from build123d import *

# Parameters (mm, degrees)
BOSS_EXTRUDE1_DEPTH = 8


with BuildPart() as part:
    # Sketch1 → Boss-Extrude1 (new body)
    with BuildSketch(Plane(origin=(0, 0, 0), x_dir=(1, 0, 0), z_dir=(0, 1, 0))):
        with BuildLine():
            Line((0, 0), (38, 0))
            ThreePointArc((38, 0), (40.636038969, 6.363961031), (47, 9))
            Line((47, 9), (99, 9))
            ThreePointArc((99, 9), (105.363961031, 6.363961031), (108, 0))
            Line((108, 0), (142, 0))
            Line((142, 0), (172.50354814, 93.880267937))
            ThreePointArc((172.50354814, 93.880267937), (166.569139078, 124.354715336), (137.573015724, 135.451290736))
            Line((137.573015724, 135.451290736), (79.487889635, 127.207214423))
            Line((79.487889635, 127.207214423), (0, 0))
        make_face()
        with BuildLine():
            Line((97.109133521, 75.428206388), (131.785075785, 80.179945877))
            ThreePointArc((131.785075785, 80.179945877), (139.670612135, 74.195105322), (133.68577158, 66.309568971))
            Line((133.68577158, 66.309568971), (99.009829317, 61.557829483))
            ThreePointArc((99.009829317, 61.557829483), (95.579909698, 60.235342824), (93.103530342, 57.518568112))
            ThreePointArc((93.103530342, 57.518568112), (61.402056741, 63.469750476), (90.33394504, 77.729688746))
            ThreePointArc((90.33394504, 77.729688746), (93.449886138, 75.779245046), (97.109133521, 75.428206388))
        make_face(mode=Mode.SUBTRACT)
    extrude(amount=BOSS_EXTRUDE1_DEPTH)


solid = part.part
Check sheet for the modelled part. Datum: model origin and axes. Units: mm. A direction names the side the tool comes from. Round coordinates to 2 decimals unless told otherwise and drop trailing zeros. Order: outer loops, then holes, each group sorted by start corner. A loop starts at its lowest first (then second) coordinate and runs counter-clockwise, first axis right, second up. Notation, with made-up numbers: M -23.75,80.25 L -12.75,80.25 A24 ccw -12.75,90.25 Z; hole C 22.25,-14 d3. An arc over 180 degrees is marked long. One line per item, written item: value. Start each with the question number.
1. Section check B-B on y = 4.25. Enter the section's corners in (x, z).
2. Gauge pin test, flat ends, axial feed: P1, Ø1.5, axis at x = 154.5, y = 3, coming from the -Z side; P2, Ø3, axis at y = 1.5, z = -80, coming from the -X side; P3, Ø2, axis at y = 2, z = -113.5, coming from the +X side. Record the tip position at first contact, or that the pin passes through.
3. Section check A-A on x = 120. Enter the section's corners in (y, z) (3 decimals).
4. Scan lines: line 1 along X through (y, z) = (2.75, -8); line 2 along Z through (x, y) = (121.5, 3.5); line 3 along X through (y, z) = (5.75, -6.5). Record each from-to range of solid material in increasing order.
5. Section check C-C on x = 74.5. Enter the section's corners in (y, z).
6. Access from +Z, -Z, +X, -X, +Y, -Y to the whole of each face (thin tool, end or side, straight path). Record for faces 1 (the cylindrical face through (40.566, 3.944, -6.294)), 2 (the flat face through (125, 4, 0)), 3 (the cylindrical face through (95.623, 3.944, -60.265)).
7. Release check for a two-part mould opening along Z. For faces 4 (the flat face through (105, 0, -54)), 5 (the cylindrical face through (93.401, 3.944, -75.796)), 6 (the flat face through (19, 4, 0)) record: released by +Z, released by -Z, zero draft, split by the parting line, or undercut.
8. Section check D-D on z = -16. Enter the section's corners in (x, y), and give its area (3 significant figures).
Results found:
1. outline: M 0,0 L 79.49,-127.21 L 137.57,-135.45 A32 ccw 172.5,-93.88 L 142,0 L 108,0 A9 cw 99,-9 L 47,-9 A9 cw 38,0 Z; hole M 90.33,-77.73 A8 cw 97.11,-75.43 L 131.79,-80.18 A7 ccw 133.69,-66.31 L 99.01,-61.56 A8 cw 93.1,-57.52 A17 ccw long Z
2. P1: z = -133.56
2. P2: x = 49.05
2. P3: x = 172.86
3. outline: M 0,-132.957 L 8,-132.957 L 8,-78.565 L 0,-78.565 Z; M 0,-64.434 L 8,-64.434 L 8,0 L 0,0 Z
4. line 1: 5 to 42.88, 103.12 to 144.6
4. line 2: -133.17 to -78.77, -64.64 to 0
4. line 3: 4.06 to 40.78, 105.22 to 144.11
5. outline: M 0,-119.22 L 8,-119.22 L 8,-82.36 L 0,-82.36 Z; M 0,-49.2 L 8,-49.2 L 8,-9 L 0,-9 Z
6. face 1: +Z, +Y, -Y
6. face 2: +Z, +X, -X, +Y, -Y
6. face 3: +Y, -Y
7. face 4: zero draft
7. face 5: undercut
7. face 6: released by +Z
8. outline: M 10,0 L 147.2,0 L 147.2,8 L 10,8 Z
8. area: 1,100 mm^2
